Verification items for the finished model (mm, model axes). A direction names the side the tool comes from. Round coordinates to 2 decimals unless told otherwise and drop trailing zeros. Order: outer loops, then holes, each group sorted by start corner. A loop starts at its lowest first (then second) coordinate and runs counter-clockwise, first axis right, second up. Notation, with made-up numbers: (-36, 55.5) -> (-15, 55.5) arc R13 ccw to (-15, 69.5) -> close; hole circle Ø8 at (27, -37.75). An arc over 180 degrees is marked (long way). Return JSON: item names as keys, results as strings. Group by question number.
Item 1: Draft check along Y on faces 1 (the cylindrical face through (31.988, 16.099, 12.325)), 2 (the flat face through (-55, 5, 70)), 3 (the flat face through (-51, 20, 58)). Enter one of: pulls with the +Y half, pulls with the -Y half, needs draft (parallel to the pull), parting line crosses it, or undercut.
Item 2: Scan lines: probe 1 along Y at (x, z) = (-46, 50); probe 2 along Z at (x, y) = (2, 43); probe 3 along Z at (x, y) = (23, 28). Record each from-to range of solid material in increasing order. Write a range as from..to.
Item 3: Access from +Z, -Z, +X, -X, +Y, -Y to the whole of each face (thin tool, end or side, straight path). Record for faces 4 (the flat face through (21, 0, 23)), 5 (the flat face through (-49, 15, 46)), 6 (the flat face through (0, 15, 28)).
Item 4: Sectioned sample at D-D on z = 9. Record the cut outline in (x, y), plus the area to 3 significant figures.
Item 5: Sectioned sample at B-B on z = 22. Record the cut outline in (x, y).
Item 6: Depth check by flat-ended pin: pin 1 Ø1.5 at (y, z) = (-2.5, 56) entering from +X; pin 2 Ø4 at (x, z) = (17.5, 23) entering from -Y; pin 3 Ø20.5 at (x, z) = (-26, 43) entering from +Y; pin 4 Ø12.5 at (y, z) = (19, 10.5) entering from -X. Enter the tip coordinate at first touch or a pass-through.
Item 7: Sectioned sample at A-A on y = 15. Record the cut outline in (x, z).
Item 8: Sectioned sample at C-C on x = -25. Record the cut outline in (y, z), plus the area to 3 significant figures.
Solid Edge part; units mm, degrees
sketch "Sketch1" plane through (0, 0, 0) normal (0, -1, 0) x (1, 0, 0)
  line L0 (-40, 70) -> (-70, 70)
  arc A0 (-70, 70) -> (0, 0) centre (0, 70) ccw
  line L1 (0, 30) -> (0, 0)
  arc A1 (-40, 70) -> (0, 30) centre (0, 70) ccw
extrude "Protrusion1" add sketch "Sketch1" against normal blind 30
sketch "Sketch2" plane through (-27.4086, 15, 70) normal (0, 0, 1) x (1, 0, 0)
  line L0 (7.4086, -5) -> (-42.5914, -5)
  line L1 (-42.5914, -5) -> (-42.5914, 5)
  line L2 (-42.5914, 5) -> (7.4086, 5)
  line L3 (7.4086, 5) -> (7.4086, -5)
extrude "ExtrudedCutout_4" cut sketch "Sketch2" against normal blind 24
sketch "Sketch3" plane through (0, 0, 0) normal (0, 0, 1) x (1, 0, 0)
  line L0 (-18, 65) -> (-18, -35)
  arc A0 (-18, 65) -> (-18, -35) centre (-18, 15) cw
extrude "ExtrudedProtrusion_2" add sketch "Sketch3" along normal blind 25
sketch "Sketch4" plane through (7, 15, 25) normal (0, 0, 1) x (0, 1, 0)
  line L0 (-15, -4.697) -> (15, -4.697)
  line L1 (15, -4.697) -> (15, -22.697)
  arc A0 (-15, -22.697) -> (15, -22.697) centre (0, 25) ccw
  line L2 (-15, -22.697) -> (-15, -4.697)
extrude "ExtrudedCutout_5" cut sketch "Sketch4" against normal blind 5
Recorded:
{
 "1": {"face 1": "parting line crosses it", "face 2": "needs draft", "face 3": "undercut"},
 "2": {"probe 1": "0..10, 20..30", "probe 2": "0..25", "probe 3": "0..20"},
 "3": {"face 4": "+Z, +X", "face 5": "+Z, +X, -X", "face 6": "+Z, +X, +Y, -Y"},
 "4": {"outline": "(-34.34, 0) -> (-18, 0) -> (-18, -35) arc R50 ccw to (-18, 65) -> (-18, 30) -> (-34.34, 30) -> close", "area": "4,420 mm²"},
 "5": {"outline": "(-50.95, 0) -> (-18, 0) -> (-18, -35) arc R50 ccw to (29.7, 0) -> (11.7, 0) -> (11.7, 30) -> (29.7, 30) arc R50 ccw to (-18, 65) -> (-18, 30) -> (-50.95, 30) -> close"},
 "6": {"pin 1": "through", "pin 2": "y = -22.12", "pin 3": "y = 30", "pin 4": "x = -45.44"},
 "7": {"outline": "(-65.76, 46) arc R70 ccw to (-18, 2.35) -> (-18, 0) -> (32, 0) -> (32, 20) -> (11.7, 20) -> (11.7, 25) -> (0, 25) -> (0, 30) arc R40 cw to (-32, 46) -> close"},
 "8": {"outline": "(0, 4.62) -> (30, 4.62) -> (30, 38.78) -> (0, 38.78) -> close", "area": "1,020 mm²"}
}
